Here's how the part is built. I have some questions about the finished solid (model axes, mm). Coordinates: 2 decimals unless noted, no trailing zeros. Write each loop counter-clockwise with the first axis right and the second up, starting at its lowest first coordinate (ties: lowest second). Pieces come first, ordered by that corner, then holes. Notation, with made-up numbers: (-11, 42.5) -> (16, 42.5) arc R28 cw to (16, 66.5) -> close; hole circle Ø4 at (45, 22.5). An arc over 180 degrees is marked (long way). Put each result on its own line as item: value. Start each with the question number.
Item 1: I want a section at C-C, the plane x = 43. List the corners of the cut face in (y, z) for me, then the cut area to 3 significant figures.
Item 2: I want a section at B-B, the plane y = 12.5. List the corners of the cut face in (x, z) for me, then the cut area to 3 significant figures.
Item 3: For pin 1 (1.9 mm diameter, centred on x = 43, y = 20.5, fed in from +Z); pin 2 (3 mm diameter, centred on y = 39, z = 5.5, fed in from +X); pin 3 (3.5 mm diameter, centred on x = 35, y = 12.5, fed in from +Z), each with a flat end and sliding along its axis, tell me the tip position at first contact or that it passes through.
Item 4: I need wall thicknesses on line 1 (Y direction, x = 43, z = 0.8); line 2 (Z direction, x = 29, y = 2); line 3 (Y direction, x = 20.25, z = 5). Which ranges of each line are inside material? Lowest first, please. Write a range as [from, to].
Item 5: I want a section at A-A, the plane x = 35. List the corners of the cut face in (y, z) for me, then the cut area to 3 significant figures.
Item 6: I want a section at D-D, the plane y = 28. List the corners of the cut face in (x, z) for me.
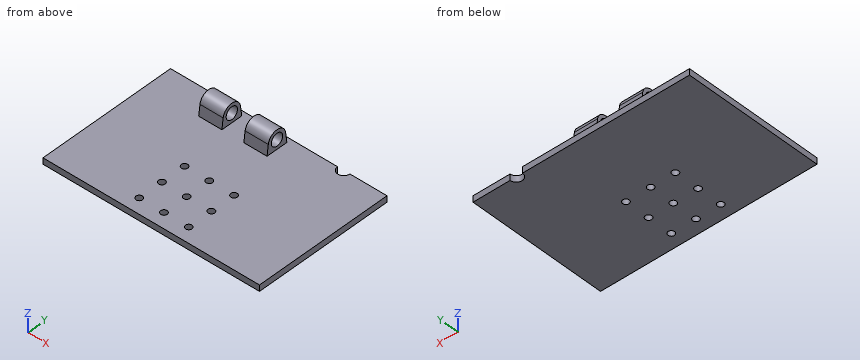
from build123d import *

# Parameters (mm, degrees)
SKETCH2_W           = 70
SKETCH2_H           = 45
BOSS_EXTRUDE1_DEPTH = 2
SKETCH3_R           = 1.05
CUT_EXTRUDE1_DEPTH  = 2
SKETCH6_R           = 2
BOSS_EXTRUDE2_DEPTH = 7.5
SKETCH4_R           = 2
CUT_EXTRUDE2_DEPTH  = 10


with BuildPart() as part:
    # Sketch2 → Boss-Extrude1 (new body)
    with BuildSketch(Plane.XY):
        with Locations((35, 22.5)):
            Rectangle(SKETCH2_W, SKETCH2_H)
    extrude(amount=BOSS_EXTRUDE1_DEPTH)

    # Sketch3 → Cut-Extrude1 (cut)
    with BuildSketch(Plane.XY.offset(2)):
        with Locations((35, 4.5)):
            Circle(SKETCH3_R)
        with Locations((43, 4.5)):
            Circle(SKETCH3_R)
        with Locations((27, 4.5)):
            Circle(SKETCH3_R)
        with Locations((27, 12.5)):
            Circle(SKETCH3_R)
        with Locations((35, 12.5)):
            Circle(SKETCH3_R)
        with Locations((43, 12.5)):
            Circle(SKETCH3_R)
        with Locations((27, 20.5)):
            Circle(SKETCH3_R)
        with Locations((35, 20.5)):
            Circle(SKETCH3_R)
        with Locations((43, 20.5)):
            Circle(SKETCH3_R)
    extrude(amount=-CUT_EXTRUDE1_DEPTH, mode=Mode.SUBTRACT)

    # Sketch6 → Boss-Extrude2 (add)
    with BuildSketch(Plane.ZY.offset(-16.9)):
        with BuildLine():
            Line((2, 43.5), (2, 36.5))
            Line((2, 36.5), (5.400666216, 36.946171815))
            ThreePointArc((5.400666216, 36.946171815), (8.08, 40), (5.400666216, 43.053828185))
            Line((5.400666216, 43.053828185), (2, 43.5))
        make_face()
        with Locations((5, 40)):
            Circle(SKETCH6_R, mode=Mode.SUBTRACT)
    boss_extrude2 = extrude(amount=-BOSS_EXTRUDE2_DEPTH)

    # Mirror4: Boss-Extrude2 across plane
    add(boss_extrude2.mirror(Plane(origin=(27.95, 0, 0), x_dir=(0, 0, 1), z_dir=(1, 0, 0))))

    # Sketch4 → Cut-Extrude2 (cut)
    with BuildSketch(Plane.XY.offset(2)):
        with Locations((56, 45)):
            Circle(SKETCH4_R)
    extrude(amount=-CUT_EXTRUDE2_DEPTH, mode=Mode.SUBTRACT)


solid = part.part
Calculated:
1. outline: (0, 0) -> (3.45, 0) -> (3.45, 2) -> (0, 2) -> close; (5.55, 0) -> (11.45, 0) -> (11.45, 2) -> (5.55, 2) -> close; (13.55, 0) -> (19.45, 0) -> (19.45, 2) -> (13.55, 2) -> close; (21.55, 0) -> (45, 0) -> (45, 2) -> (21.55, 2) -> close
1. area: 77.4 mm2
2. outline: (0, 0) -> (25.95, 0) -> (25.95, 2) -> (0, 2) -> close; (28.05, 0) -> (33.95, 0) -> (33.95, 2) -> (28.05, 2) -> close; (36.05, 0) -> (41.95, 0) -> (41.95, 2) -> (36.05, 2) -> close; (44.05, 0) -> (70, 0) -> (70, 2) -> (44.05, 2) -> close
2. area: 127 mm2
3. pin 1: passes through
3. pin 2: stops at x = 39
3. pin 3: stops at z = 2
4. line 1: y = [0, 3.45], [5.55, 11.45], [13.55, 19.45], [21.55, 45]
4. line 2: z = [0, 2]
4. line 3: y = [36.89, 38], [42, 43.11]
5. outline: (0, 0) -> (3.45, 0) -> (3.45, 2) -> (0, 2) -> close; (5.55, 0) -> (11.45, 0) -> (11.45, 2) -> (5.55, 2) -> close; (13.55, 0) -> (19.45, 0) -> (19.45, 2) -> (13.55, 2) -> close; (21.55, 0) -> (45, 0) -> (45, 2) -> (43.5, 2) -> (43.05, 5.4) arc R3.08 ccw to (36.95, 5.4) -> (36.5, 2) -> (21.55, 2) -> close; hole circle Ø4 at (40, 5)
5. area: 99.6 mm2
6. outline: (0, 0) -> (70, 0) -> (70, 2) -> (0, 2) -> close
